Autodesk Inventor part; units mm, degrees
ref_plane "YZ Plane" through (0, 0, 0) normal (1, 0, 0) x (0, 1, 0)
ref_plane "XZ Plane" through (0, 0, 0) normal (0, 1, 0) x (-1, 0, 0)
ref_plane "XY Plane" through (0, 0, 0) normal (0, 0, 1) x (1, 0, 0)
sketch "Sketch1" plane through (0, 0, 0) normal (0, 1, 0) x (-1, 0, 0)
  line L0 (0, 0) -> (40, 0)
  line L1 (40, 0) -> (40, -150)
  line L2 (40, -150) -> (0, -150)
  line L3 (0, -150) -> (0, 0)
  dimension "d0" = 40
  dimension "d1" = 150
extrude "Extrusion1" add sketch "Sketch1" along normal blind 5
sketch "Sketch2" plane through (0, 5, 0) normal (0, 1, 0) x (1, 0, 0)
  line L0 (-40, 0) -> (0, 0)
  line L1 (0, 150) -> (-40, 150)
  line L2 (-40, 0) -> (-20, 0)
  line L3 (-20, 0) -> (-20, 150)
  line L4 (-20, 150) -> (-40, 150)
  line L5 (-40, 150) -> (-40, 0)
  line L6 (-20, 0) -> (-20, 75)
  line L7 (-20, 75) -> (-20, 35)
  line L8 (-20, 35) -> (-28, 35)
  line L9 (-28, 35) -> (-28, 25)
  line L10 (-28, 25) -> (-20, 25)
  line L11 (-20, 25) -> (-20, 35)
  line L12 (-20, 25) -> (-12, 25)
  line L13 (-12, 25) -> (-12, 35)
  line L14 (-12, 35) -> (-20, 35)
  line L15 (-20, 35) -> (-20, 25)
  line L16 (-20, 75) -> (-20, 115)
  line L17 (-20, 115) -> (-28, 115)
  line L18 (-28, 115) -> (-28, 125)
  line L19 (-28, 125) -> (-20, 125)
  line L20 (-20, 125) -> (-20, 115)
  line L21 (-20, 115) -> (-12, 115)
  line L22 (-12, 115) -> (-12, 125)
  line L23 (-12, 125) -> (-20, 125)
  line L24 (-20, 125) -> (-20, 115)
  line L25 (-28, 125) -> (-12, 125)
  line L26 (-12, 125) -> (-12, 25)
  line L27 (-12, 25) -> (-28, 25)
  line L28 (-28, 25) -> (-28, 125)
  dimension "d4" = 75
  dimension "d5" = 40
  dimension "d6" = 8
  dimension "d7" = 10
  dimension "d8" = 8
  dimension "d9" = 40
  dimension "d10" = 10
extrude "Extrusion2" add sketch "Sketch2" along normal blind 25 contours L10 L9 L8 L3 | L3 L14 L13 L12 | L8 L28 L17 L3 | L3 L21 L26 L14 | L23 L22 L21 L3 | L3 L17 L18 L19
sketch "Sketch3" plane through (0, 30, 0) normal (0, 1, 0) x (1, 0, 0)
  line L0 (-12, 25) -> (-28, 25)
  line L1 (-20, 25) -> (-20, 125)
  line L2 (-12, 125) -> (-28, 125)
  line L3 (-20, 25) -> (-20, 75)
  line L4 (-20, 75) -> (-20, 35)
  line L5 (-20, 35) -> (-20, 115)
  circle A0 centre (-20, 35) radius 2
  circle A1 centre (-20, 75) radius 2
  circle A2 centre (-20, 115) radius 2
  point P0 (0, 0)
  dimension "d13" = 40
  dimension "d14" = 80
  dimension "d15" = 4
  dimension "d16" = 4
  dimension "d17" = 4
extrude "Extrusion3" cut sketch "Sketch3" against normal blind 12.5
properties part number "Pin holder"
Design review of the part built by this model. Coordinates are the model's own, in mm. A direction names the side the tool comes from. Coordinates: 2 decimals unless noted, no trailing zeros. Order: outer loops, then holes, each group sorted by start corner. A loop starts at its lowest first (then second) coordinate and runs counter-clockwise, first axis right, second up. Notation, with made-up numbers: (-26, 5) -> (-6, 5) arc R18 ccw to (-6, 30) -> close; hole circle Ø10 at (45, 16). An arc over 180 degrees is marked (long way). Use one line per item in the form item = value. Start each with the question number.
(1) Add section C-C on z = -75. State the section outline as (x, y) points, plus the area to 3 significant figures.
(2) For probe 1 along Z at (x, y) = (-20, 22); probe 2 along X at (y, z) = (21.25, -115); probe 3 along Y at (x, z) = (-2, -24), list the stretches that pass through material, from the lowest coordinate up.
(3) For faces 4 (the cylindrical face through (-20, 24, -77)), 5 (the flat face through (-12, 17, -74)), 6 (the flat face through (-20, 17, -125)), list the 3-axis set-ups (+Z, -Z, +X, -X, +Y, -Y) from which the entire face can be reached by the end or side of a thin tool; tool diameter is ignored.
(4) The part is to be moulded in two halves that separate along X. For faces 1 (the flat face through (-28, 17, -76)), 2 (the flat face through (-20, 17, -25)), 3 (the cylindrical face through (-20, 24, -33)), say which applies: +X half, -X half, draft (parallel to the pull), parting line (faces both ways), or undercut.
(5) Add section D-D on y = 14.5. State the section outline as (x, z) points.
(6) Add section A-A on y = 26.5. State the section outline as (x, z) points, plus the area to 3 significant figures.
(7) Add section B-B on x = -20. State the section outline as (y, z) points.
(8) Insertion check: pin 1 (3 mm diameter, centred on x = -20, z = -115, fed in from +Y); pin 2 (4 mm diameter, centred on y = 16, z = -84.5, fed in from +X); pin 3 (13 mm diameter, centred on x = -16, y = 16.5, fed in from -Z). Each pin has a flat end and moves straight along its axis. Give the tip position at first contact, or say it passes through.
Answer block:
q1.outline = (-40, 0) -> (0, 0) -> (0, 5) -> (-12, 5) -> (-12, 30) -> (-18, 30) -> (-18, 17.5) -> (-22, 17.5) -> (-22, 30) -> (-28, 30) -> (-28, 5) -> (-40, 5) -> close
q1.area = 550 mm²
q2.probe_1 = -125 to -117, -113 to -77, -73 to -37, -33 to -25
q2.probe_2 = -28 to -22, -18 to -12
q2.probe_3 = 0 to 5
q3.face_4 = +Y
q3.face_5 = +Z, -Z, +X, +Y
q3.face_6 = -Z, +X, -X, +Y
q4.face_1 = -X half
q4.face_2 = draft
q4.face_3 = undercut
q5.outline = (-28, -125) -> (-12, -125) -> (-12, -25) -> (-28, -25) -> close
q6.outline = (-28, -125) -> (-12, -125) -> (-12, -25) -> (-28, -25) -> close; hole circle Ø4 at (-20, -115); hole circle Ø4 at (-20, -75); hole circle Ø4 at (-20, -35)
q6.area = 1,560 mm²
q7.outline = (0, -150) -> (5, -150) -> (5, -125) -> (30, -125) -> (30, -117) -> (17.5, -117) -> (17.5, -113) -> (30, -113) -> (30, -77) -> (17.5, -77) -> (17.5, -73) -> (30, -73) -> (30, -37) -> (17.5, -37) -> (17.5, -33) -> (30, -33) -> (30, -25) -> (5, -25) -> (5, 0) -> (0, 0) -> close
q8.pin_1 = 17.5
q8.pin_2 = -12
q8.pin_3 = -125
